Autodesk Inventor part; units mm, degrees
ref_plane "YZ Plane" through (0, 0, 0) normal (1, 0, 0) x (0, 1, 0)
ref_plane "XZ Plane" through (0, 0, 0) normal (0, 1, 0) x (-1, 0, 0)
ref_plane "XY Plane" through (0, 0, 0) normal (0, 0, 1) x (1, 0, 0)
sketch "Sketch1" plane through (0, 0, 0) normal (0, 0, 1) x (1, 0, 0)
  line L0 (0, 0) -> (0, 6.5)
  line L1 (0, 6.5) -> (5.6292, 3.25)
  line L2 (0, 6.5) -> (6.5, 6.5) construction
  line L3 (5.6292, 3.25) -> (5.6292, -3.25)
  line L4 (5.6292, -3.25) -> (0, -6.5)
  line L5 (0, -6.5) -> (-5.6292, -3.25)
  line L6 (-5.6292, -3.25) -> (-5.6292, 3.25)
  line L7 (-5.6292, 3.25) -> (0, 6.5)
  circle A0 centre (0, 0) radius 3.175
  dimension "d1" = 6.5
  dimension "d2" = 30
  dimension "d3" = 6.35
extrude "Extrusion1" add sketch "Sketch1" along normal blind 25
chamfer "Chamfer1" distance 0.25 angle 45 18 edges at (2.8146, 4.875, 25) (5.6292, 0, 25) (2.8146, -4.875, 25) (-2.8146, -4.875, 25) (-5.6292, 0, 25) (-2.8146, 4.875, 25) (0, 6.5, 12.5) (5.6292, 3.25, 12.5) (5.6292, -3.25, 12.5) (0, -6.5, 12.5) (-5.6292, -3.25, 12.5) (-5.6292, 3.25, 12.5) (-2.8146, 4.875, 0) (-5.6292, 0, 0) (-2.8146, -4.875, 0) (2.8146, -4.875, 0) (5.6292, 0, 0) (2.8146, 4.875, 0)
thread "Thread1"
properties part number "5002_Brass_Nut_Tx_Rx_Relative_Positioning_MPSv2_v1" material "Brass, Soft Yellow"
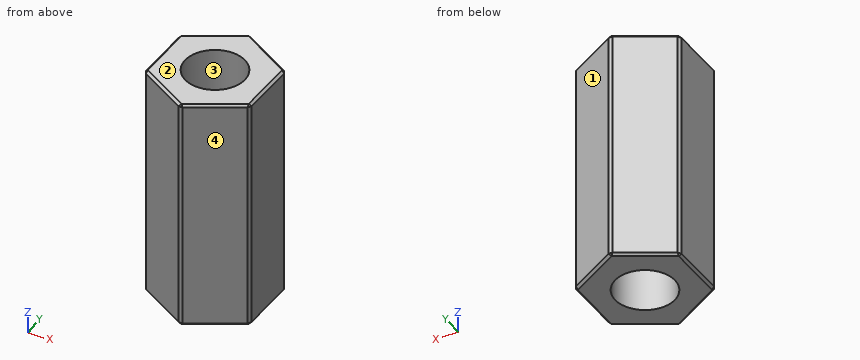
Geometry check sheet. Reference: the model listing, model coordinates, mm. Face numbers are marked on the shaded views. Give positions to 0.01 mm unless a question says otherwise; leave off trailing zeros. Order: outer loops, then holes, each group sorted by start corner. A loop starts at its lowest first (then second) coordinate and runs counter-clockwise, first axis right, second up. Notation, with made-up numbers: (6.25, -1) - (31.25, -1) arc R23 ccw to (31.25, 26) - close; hole circle Ø8 at (85.25, 39). An arc over 180 degrees is marked (long way). Answer in a Markdown table with one row per item. Add a question column.
Q1. Mould release check, pull along Y, two halves, no side actions. Record for the marked faces 1, 2, 3 and 4: pulls with the +Y half, pulls with the -Y half, needs draft (parallel to the pull), parting line crosses it, or undercut.
Q2. Cross-section at D-D, the plane x = -3.5. Enter the section's corners in (y, z), then the cut area to 3 significant figures.
Q3. Material ranges on probe 1 along X at (y, z) = (0, 13) (3 decimals); probe 2 along Y at (x, z) = (0, 9.5) (3 decimals); probe 3 along X at (y, z) = (-2, 9.5), recorded low to high. Write a range as from..to.
Q4. Cross-section at A-A, the plane y = 0. Enter the section's corners in (x, z) (3 decimals).
Q5. Gauge pin test, flat end, axial feed: pin 1 (4 mm diameter, centred on x = -3.5, z = 21.5, fed in from -Y). Record the tip position at first contact, or that the pin passes through.
Q6. Cross-section at C-C, the plane x = 0.75. Enter the section's corners in (y, z).
Check values:
| question | item | result |
|---|---|---|
| 1 | face 1 | pulls with the +Y half |
| 1 | face 2 | needs draft |
| 1 | face 3 | undercut |
| 1 | face 4 | pulls with the -Y half |
| 2 | outline | (-4.48, 0.25) - (-4.19, 0) - (4.19, 0) - (4.48, 0.25) - (4.48, 24.75) - (4.19, 25) - (-4.19, 25) - (-4.48, 24.75) - close |
| 2 | area | 224 mm^2 |
| 3 | probe 1 | x = -5.629..-3.175, 3.175..5.629 |
| 3 | probe 2 | y = -6.375..-3.175, 3.175..6.375 |
| 3 | probe 3 | x = -5.63..-2.47, 2.47..5.63 |
| 4 | outline | (-5.629, 0.25) - (-5.379, 0) - (-3.175, 0) - (-3.175, 25) - (-5.379, 25) - (-5.629, 24.75) - close; (3.175, 0) - (5.379, 0) - (5.629, 0.25) - (5.629, 24.75) - (5.379, 25) - (3.175, 25) - close |
| 5 | pin 1 | stops at y = -5.63 |
| 6 | outline | (-6.07, 0.25) - (-5.78, 0) - (-3.09, 0) - (-3.09, 25) - (-5.78, 25) - (-6.07, 24.75) - close; (3.09, 0) - (5.78, 0) - (6.07, 0.25) - (6.07, 24.75) - (5.78, 25) - (3.09, 25) - close |
